from build123d import *

# Parameters (mm, degrees)
CROQUIS1_R              = 2
CROQUIS1_R_2            = 7.5
CROQUIS1_R_3            = 17.4
CROQUIS1_R_4            = 11
CROQUIS1_R_5            = 1.5
CROQUIS1_R_6            = 3
SALIENTE_EXTRUIR1_DEPTH = 2
CROQUIS2_R              = 2
CORTAR_EXTRUIR1_DEPTH   = 10
CROQUIS3_R              = 2
CORTAR_EXTRUIR2_DEPTH   = 10
CROQUIS4_R              = 2
CORTAR_EXTRUIR3_DEPTH   = 10


with BuildPart() as part:
    # Croquis1 → Saliente-Extruir1 (new, symmetric)
    with BuildSketch(Plane.XY):
        with BuildLine():
            Line((-178.895080774, -40.856503162), (179.195612521, -40.220204958))
            Line((179.195612521, -40.220204958), (190.010789857, -40.220204958))
            ThreePointArc((190.010789857, -40.220204958), (194.944809403, -39.514865591), (199.483580997, -37.455349889))
            Line((199.483580997, -37.455349889), (272.742664287, 9.291785175))
            ThreePointArc((272.742664287, 9.291785175), (286.437106864, 39.932371901), (260, 60.607542834))
            Line((260, 60.607542834), (-260, 60.607542834))
            ThreePointArc((-260, 60.607542834), (-287.659968635, 38.976031395), (-273.332082679, 6.918148807))
            Line((-273.332082679, 6.918148807), (-188.316697637, -38.71919799))
            ThreePointArc((-188.316697637, -38.71919799), (-183.7609115, -40.471216098), (-178.895080774, -40.856503162))
        make_face()
        with Locations((0, -23.892457166)):
            Circle(CROQUIS1_R, mode=Mode.SUBTRACT)
        with Locations((-90, -23.892457166)):
            Circle(CROQUIS1_R, mode=Mode.SUBTRACT)
        with Locations((-180, -23.892457166)):
            Circle(CROQUIS1_R, mode=Mode.SUBTRACT)
        with Locations((-90, 32.107542834)):
            Circle(CROQUIS1_R_2, mode=Mode.SUBTRACT)
        with Locations((0, 32.107542834)):
            Circle(CROQUIS1_R_2, mode=Mode.SUBTRACT)
        with Locations((-260, 32.107542834)):
            Circle(CROQUIS1_R_3, mode=Mode.SUBTRACT)
        with Locations(Location((260, 33.367542834, 0), (0, 0, 180))):
            Circle(CROQUIS1_R_4, mode=Mode.SUBTRACT)
        with Locations(Location((90, 32.107542834, 0), (0, 0, 180))):
            Circle(CROQUIS1_R_2, mode=Mode.SUBTRACT)
        with Locations(Location((90, -23.892457166, 0), (0, 0, 180))):
            Circle(CROQUIS1_R, mode=Mode.SUBTRACT)
        with Locations(Location((-180, 32.107542834, 0), (0, 0, 180))):
            Circle(CROQUIS1_R_2, mode=Mode.SUBTRACT)
        with Locations((180, 32.107542834)):
            Circle(CROQUIS1_R_2, mode=Mode.SUBTRACT)
        with Locations((-8, 6.607542834)):
            Circle(CROQUIS1_R_5, mode=Mode.SUBTRACT)
        with Locations((0, 14.607542834)):
            Circle(CROQUIS1_R_5, mode=Mode.SUBTRACT)
        with Locations((8, 6.607542834)):
            Circle(CROQUIS1_R_5, mode=Mode.SUBTRACT)
        with Locations((0, -1.392457166)):
            Circle(CROQUIS1_R_5, mode=Mode.SUBTRACT)
        with Locations((0, 6.607542834)):
            Circle(CROQUIS1_R_6, mode=Mode.SUBTRACT)
        with Locations((180, -23.892457166)):
            Circle(CROQUIS1_R, mode=Mode.SUBTRACT)
        with BuildLine():
            Line((-82.5, 12.107542834), (-82.5, -3.892457166))
            ThreePointArc((-82.5, -3.892457166), (-90, -11.392457166), (-97.5, -3.892457166))
            Line((-97.5, -3.892457166), (-97.5, 12.107542834))
            ThreePointArc((-97.5, 12.107542834), (-90, 19.607542834), (-82.5, 12.107542834))
        make_face(mode=Mode.SUBTRACT)
        with BuildLine():
            Line((-20, 24.607542834), (-70, 24.607542834))
            ThreePointArc((-70, 24.607542834), (-77.5, 32.107542834), (-70, 39.607542834))
            Line((-70, 39.607542834), (-20, 39.607542834))
            ThreePointArc((-20, 39.607542834), (-12.5, 32.107542834), (-20, 24.607542834))
        make_face(mode=Mode.SUBTRACT)
        with BuildLine():
            Line((160, -26.392457166), (110, -26.392457166))
            ThreePointArc((110, -26.392457166), (102.5, -18.892457166), (110, -11.392457166))
            Line((110, -11.392457166), (160, -11.392457166))
            ThreePointArc((160, -11.392457166), (167.5, -18.892457166), (160, -26.392457166))
        make_face(mode=Mode.SUBTRACT)
        with BuildLine():
            Line((20, -11.392457166), (70, -11.392457166))
            ThreePointArc((70, -11.392457166), (77.5, -18.892457166), (70, -26.392457166))
            Line((70, -26.392457166), (20, -26.392457166))
            ThreePointArc((20, -26.392457166), (12.5, -18.892457166), (20, -11.392457166))
        make_face(mode=Mode.SUBTRACT)
        with BuildLine():
            Line((20, 39.607542834), (70, 39.607542834))
            ThreePointArc((70, 39.607542834), (77.5, 32.107542834), (70, 24.607542834))
            Line((70, 24.607542834), (20, 24.607542834))
            ThreePointArc((20, 24.607542834), (12.5, 32.107542834), (20, 39.607542834))
        make_face(mode=Mode.SUBTRACT)
        with BuildLine():
            Line((-160, 39.607542834), (-110, 39.607542834))
            ThreePointArc((-110, 39.607542834), (-102.5, 32.107542834), (-110, 24.607542834))
            Line((-110, 24.607542834), (-160, 24.607542834))
            ThreePointArc((-160, 24.607542834), (-167.5, 32.107542834), (-160, 39.607542834))
        make_face(mode=Mode.SUBTRACT)
        with BuildLine():
            Line((-20, -26.392457166), (-70, -26.392457166))
            ThreePointArc((-70, -26.392457166), (-77.5, -18.892457166), (-70, -11.392457166))
            Line((-70, -11.392457166), (-20, -11.392457166))
            ThreePointArc((-20, -11.392457166), (-12.5, -18.892457166), (-20, -26.392457166))
        make_face(mode=Mode.SUBTRACT)
        with BuildLine():
            Line((160, 24.607542834), (110, 24.607542834))
            ThreePointArc((110, 24.607542834), (102.5, 32.107542834), (110, 39.607542834))
            Line((110, 39.607542834), (160, 39.607542834))
            ThreePointArc((160, 39.607542834), (167.5, 32.107542834), (160, 24.607542834))
        make_face(mode=Mode.SUBTRACT)
        with BuildLine():
            Line((-160, -26.392457166), (-110, -26.392457166))
            ThreePointArc((-110, -26.392457166), (-102.5, -18.892457166), (-110, -11.392457166))
            Line((-110, -11.392457166), (-160, -11.392457166))
            ThreePointArc((-160, -11.392457166), (-167.5, -18.892457166), (-160, -26.392457166))
        make_face(mode=Mode.SUBTRACT)
        with BuildLine():
            Line((97.5, 12.107542834), (97.5, -3.892457166))
            ThreePointArc((97.5, -3.892457166), (90, -11.392457166), (82.5, -3.892457166))
            Line((82.5, -3.892457166), (82.5, 12.107542834))
            ThreePointArc((82.5, 12.107542834), (90, 19.607542834), (97.5, 12.107542834))
        make_face(mode=Mode.SUBTRACT)
    extrude(amount=SALIENTE_EXTRUIR1_DEPTH, both=True)

    # Croquis2 → Cortar-Extruir1 (cut)
    with BuildSketch(Plane.XY.offset(2)):
        with Locations((-283.74, 32.107542834)):
            Circle(CROQUIS2_R)
        with Locations((-271.95, 52.805549985)):
            Circle(CROQUIS2_R)
        with Locations((-248.05, 52.805549985)):
            Circle(CROQUIS2_R)
        with Locations((-236.1, 32.107542834)):
            Circle(CROQUIS2_R)
        with Locations((-248.05, 11.409535684)):
            Circle(CROQUIS2_R)
        with Locations((-271.95, 11.409535684)):
            Circle(CROQUIS2_R)
    extrude(amount=-CORTAR_EXTRUIR1_DEPTH, mode=Mode.SUBTRACT)

    # Croquis3 → Cortar-Extruir2 (cut)
    with BuildSketch(Plane.XY.offset(2)):
        with Locations((260, 51.367542834)):
            Circle(CROQUIS3_R)
        with Locations((275.588457268, 42.367542834)):
            Circle(CROQUIS3_R)
        with Locations((275.588457268, 24.367542834)):
            Circle(CROQUIS3_R)
        with Locations((260, 15.367542834)):
            Circle(CROQUIS3_R)
        with Locations((244.411542732, 24.367542834)):
            Circle(CROQUIS3_R)
        with Locations((244.411542732, 42.367542834)):
            Circle(CROQUIS3_R)
    extrude(amount=-CORTAR_EXTRUIR2_DEPTH, mode=Mode.SUBTRACT)

    # Croquis4 → Cortar-Extruir3 (cut)
    with BuildSketch(Plane.XY.offset(2)):
        with Locations((-157.256763594, 48.107542834)):
            Circle(CROQUIS4_R)
        with Locations((-67.256763594, 48.107542834)):
            Circle(CROQUIS4_R)
        with Locations((22.743236406, 48.107542834)):
            Circle(CROQUIS4_R)
        with Locations((112.743236406, 48.107542834)):
            Circle(CROQUIS4_R)
        with Locations((202.743236406, 48.107542834)):
            Circle(CROQUIS4_R)
    extrude(amount=-CORTAR_EXTRUIR3_DEPTH, mode=Mode.SUBTRACT)


solid = part.part
The listing builds one solid part. Answer for the finished solid, in the listing's coordinates (mm). Round coordinates to 2 decimals unless told otherwise and drop trailing zeros. Write each loop counter-clockwise with the first axis right and the second up, starting at its lowest first coordinate (ties: lowest second). Pieces come first, ordered by that corner, then holes. Notation, with made-up numbers: M 75.25,58.25 L 133.25,58.25 A3 ccw 133.25,63.25 Z; hole C -22,6.25 d1. An arc over 180 degrees is marked long. Write each question's results on one line, items separated by ' | '. Start each with the question number.
Item 1: Find section D-D on x = 212. Write down the section's boundary in (y, z).
Item 2: Given pin 1 Ø8 at (x, y) = (-23.5, -21.5) entering from -Z; pin 2 Ø2 at (x, z) = (-143, -0.5) entering from -Y; pin 3 Ø2 at (y, z) = (7.5, 0) entering from -X; pin 4 Ø1 at (y, z) = (-13.5, -1.5) entering from +X, each flat-ended and moving along its own axis, determine where each tip first touches the part or whether it passes through.
Item 3: Find section B-B on y = -17. Write down the section's boundary in (x, z).
Item 4: Find section A-A on x = -135.5. Write down the section's boundary in (y, z).
Item 5: The mould has two halves that part along Y. Classify faces 1 (the cylindrical face through (-287.528, 39.489, 0.028)), 2 (the flat face through (-5, 11, -2)), 3 (the cylindrical face through (-1.626, 24.786, -0.028)): +Y half, -Y half, draft (parallel to the pull), parting line (faces both ways), or undercut.
Item 6: Find section C-C on z = 1.05. Give the number of separate pieces and of enclosed holes in the cut face, and give its area (3 significant figures).
Item 7: Straight lines are drawn through the part: probe 1 along X at (y, z) = (10, -0.8); probe 2 along Y at (x, z) = (0, 0.05); probe 3 along X at (y, z) = (41.5, 0.2). For each, find the intervals that lie inside material, in ascending order.
Answer block:
1) outline: M -29.47,-2 L 60.61,-2 L 60.61,2 L -29.47,2 Z
2) pin 1: passes through | pin 2: stops at y = -40.79 | pin 3: stops at x = -275.97 | pin 4: stops at x = 237.81
3) outline: M -228.78,-2 L -167.26,-2 L -167.26,2 L -228.78,2 Z; M -102.74,-2 L -77.26,-2 L -77.26,2 L -102.74,2 Z; M -12.74,-2 L 12.74,-2 L 12.74,2 L -12.74,2 Z; M 77.26,-2 L 102.74,-2 L 102.74,2 L 77.26,2 Z; M 167.26,-2 L 231.54,-2 L 231.54,2 L 167.26,2 Z
4) outline: M -40.78,-2 L -26.39,-2 L -26.39,2 L -40.78,2 Z; M -11.39,-2 L 24.61,-2 L 24.61,2 L -11.39,2 Z; M 39.61,-2 L 60.61,-2 L 60.61,2 L 39.61,2 Z
5) face 1: parting line | face 2: draft | face 3: undercut
6) separate pieces: 1 | enclosed holes: 44 | area: 41,400 mm²
7) probe 1: x = -277.99 to -273.37, -270.53 to -249.47, -246.63 to -97.5, -82.5 to 82.5, 97.5 to 274 | probe 2: y = -40.54 to -25.89, -21.89 to -2.89, 0.11 to 3.61, 9.61 to 13.11, 16.11 to 24.61, 39.61 to 60.61 | probe 3: x = -286.91 to -274.65, -245.35 to 242.61, 246.21 to 252.59, 267.41 to 273.79, 277.39 to 286
